Source: CAD feature listing. Evaluate the final solid. Frame: model axes, mm. A direction names the side the tool comes from. Coordinates: 2 decimals unless noted, no trailing zeros. Write each loop counter-clockwise with the first axis right and the second up, starting at its lowest first coordinate (ties: lowest second). Pieces come first, ordered by that corner, then holes. Notation, with made-up numbers: M 86,49 L 123,49 A24 ccw 123,64 Z; hole C 27.5,15 d2. An arc over 180 degrees is marked long. One line per item, written item: value. Start each with the question number.
Item 1: Cut plane B-B, the plane z = 39. Output: boundary loops of the cut face in (x, y) (3 decimals), then the cut area to 3 significant figures.
Item 2: Ray query, L1, parallel to X at y = 44, z = 7.5 (1 decimal); L2, parallel to X at y = 31, z = 8 (1 decimal); L3, parallel to Y at x = 54.5, z = 28.5 (3 decimals). Return the intervals inside material, ascending. Write a range as from..to.
Item 3: Mould query, pull axis X, two halves, no side actions, for faces 3 (the flat face through (54.153, 67, 8)), 4 (the flat face through (72.758, 93.034, -1.212)), 5 (the flat face through (31.75, 96, 20)). Classes: released by +X, released by -X, zero draft, split by the parting line, or undercut.
Item 4: Cut plane C-C, the plane y = 11. Output: boundary loops of the cut face in (x, z) (1 decimal), then the cut area to 3 significant figures.
Item 5: Pin query (flat end, axial travel): P1, Ø21.5, axis at x = 25.5, z = 22, coming from the +Y side; P2, Ø5, axis at x = 13.5, z = 26, coming from the -Y side; P3, Ø0.5, axis at x = 8, y = 82.5, coming from the +Z side; P4, Ø12, axis at x = 35, z = 4.5, coming from the +Y side (3 decimals). Return the tip coordinate at first contact, or that it passes through.
Item 6: Set-up query: faces 1 (the flat face through (54.4, 72.4, 15.24)), 2 (the cylindrical face through (37.591, 103.504, 19.678)). Return all of +Z, -Z, +X, -X, +Y, -Y with unobstructed straight access to the full face (end or side cutting, diameter ignored); none if empty.
Item 7: Cut plane D-D, the plane y = 46.5. Output: boundary loops of the cut face in (x, z) (1 decimal).
```python
from build123d import *

# Parameters (mm, degrees)
SKETCH1_R           = 2.54
BOSS_EXTRUDE1_DEPTH = 3.175
SKETCH1_3_W         = 13.97
SKETCH1_3_H         = 1.5875
BOSS_EXTRUDE2_DEPTH = 10.16
SKETCH1_4_R         = 2.54
BOSS_EXTRUDE3_DEPTH = 43.18
SKETCH2_W           = 13.97
SKETCH2_H           = 1.5875
BOSS_EXTRUDE4_DEPTH = 15.24
SKETCH3_R           = 8.255
CUT_EXTRUDE1_DEPTH  = 15.24
CHAMFER1_SIZE       = 3.175


with BuildPart() as part:
    # Sketch1 → Boss-Extrude1 (new body)
    with BuildSketch(Plane.XY):
        with BuildLine():
            Line((0, 0), (31.75, 0))
            Line((31.75, 0), (31.75, -2.54))
            ThreePointArc((31.75, -2.54), (37.465, -8.255), (43.18, -2.54))
            Line((43.18, -2.54), (43.18, 0))
            Line((43.18, 0), (74.93, 0))
            Line((74.93, 0), (74.93, 95.25))
            Line((74.93, 95.25), (43.18, 95.25))
            Line((43.18, 95.25), (43.18, 97.79))
            ThreePointArc((43.18, 97.79), (37.465, 103.505), (31.75, 97.79))
            Line((31.75, 97.79), (31.75, 95.25))
            Line((31.75, 95.25), (0, 95.25))
            Line((0, 95.25), (0, 0))
        make_face()
        with Locations((37.465, -2.54)):
            Circle(SKETCH1_R, mode=Mode.SUBTRACT)
        with Locations((37.465, 97.79)):
            Circle(SKETCH1_R, mode=Mode.SUBTRACT)
    extrude(amount=-BOSS_EXTRUDE1_DEPTH)

    # Sketch1_3 → Boss-Extrude2 (add)
    with BuildSketch(Plane.XY):
        Polygon((43.815, 9.525), (43.815, 75.5015), (29.845, 75.5015), (29.845, 77.089), (43.815, 77.089), (45.4025, 77.089), (45.4025, 3.175), (43.815, 3.175), (43.815, 7.9375), (3.175, 7.9375), (3.175, 9.525), align=None)
        with Locations((10.16, 76.29525)):
            Rectangle(SKETCH1_3_W, SKETCH1_3_H)
    extrude(amount=BOSS_EXTRUDE2_DEPTH)

    # Sketch1_4 → Boss-Extrude3 (add)
    with BuildSketch(Plane.XY):
        with BuildLine():
            Line((0, 95.25), (0, 0))
            Line((0, 0), (31.75, 0))
            Line((31.75, 0), (31.75, -2.54))
            ThreePointArc((31.75, -2.54), (37.465, -8.255), (43.18, -2.54))
            Line((43.18, -2.54), (43.18, 0))
            Line((43.18, 0), (74.93, 0))
            Line((74.93, 0), (74.93, 95.25))
            Line((74.93, 95.25), (43.18, 95.25))
            Line((43.18, 95.25), (43.18, 97.79))
            ThreePointArc((43.18, 97.79), (37.465, 103.505), (31.75, 97.79))
            Line((31.75, 97.79), (31.75, 95.25))
            Line((31.75, 95.25), (0, 95.25))
        make_face()
        with Locations((37.465, -2.54)):
            Circle(SKETCH1_4_R, mode=Mode.SUBTRACT)
        Polygon((3.175, 7.9375), (3.175, 9.525), (3.175, 75.5015), (3.175, 77.089), (3.175, 92.075), (71.755, 92.075), (71.755, 3.175), (45.4025, 3.175), (43.815, 3.175), (3.175, 3.175), align=None, mode=Mode.SUBTRACT)
        with Locations((37.465, 97.79)):
            Circle(SKETCH1_4_R, mode=Mode.SUBTRACT)
    extrude(amount=BOSS_EXTRUDE3_DEPTH)

    # Sketch2 → Boss-Extrude4 (add)
    with BuildSketch(Plane.XY):
        with Locations((10.16, 82.20075)):
            Rectangle(SKETCH2_W, SKETCH2_H)
        Polygon((54.737, 82.9945), (55.740027204, 82.9945), (55.740027204, 52.60975), (54.152527204, 52.60975), (54.152527204, 81.407), (29.845, 81.407), (29.845, 82.9945), align=None)
        Polygon((54.152527204, 3.175), (55.740027204, 3.175), (55.740027204, 33.55975), (54.152527204, 33.55975), (54.152527204, 9.525), (3.175, 9.525), (3.175, 7.9375), (54.152527204, 7.9375), align=None)
    extrude(amount=BOSS_EXTRUDE4_DEPTH)

    # Sketch3 → Cut-Extrude1 (cut)
    with BuildSketch(Plane.ZY.offset(-71.755)):
        with Locations((27.1145, 13.462)):
            Circle(SKETCH3_R)
    extrude(amount=-CUT_EXTRUDE1_DEPTH, mode=Mode.SUBTRACT)

    # Chamfer1
    chamfer1_edges = [part.edges().sort_by_distance(p)[0] for p in [
        (0, 0, 20.0025),
        (0, 95.25, 20.0025),
        (59.055, 0, -3.175),
        (74.93, 95.25, 20.0025),
        (74.93, 0, 20.0025),
        (74.93, 47.625, -3.175),
        (59.055, 95.25, -3.175),
        (15.875, 95.25, -3.175),
        (0, 47.625, -3.175),
        (15.875, 0, -3.175),
    ]]
    chamfer(chamfer1_edges, length=CHAMFER1_SIZE)


solid = part.part
```
From the geometry:
1. outline: M 0,3.175 L 3.175,0 L 31.75,0 L 31.75,-2.54 A5.715 ccw 43.18,-2.54 L 43.18,0 L 71.755,0 L 74.93,3.175 L 74.93,92.075 L 71.755,95.25 L 43.18,95.25 L 43.18,97.79 A5.715 ccw 31.75,97.79 L 31.75,95.25 L 3.175,95.25 L 0,92.075 Z; hole M 3.175,3.175 L 71.755,3.175 L 71.755,92.075 L 3.175,92.075 Z; hole C 37.465,-2.54 d5.08; hole C 37.465,97.79 d5.08
1. area: 1,140 mm²
2. L1: x = 0..3.2, 43.8..45.4, 71.8..74.9
2. L2: x = 0..3.2, 43.8..45.4, 54.2..55.7, 71.8..74.9
2. L3: y = 0..3.175, 92.075..95.25
3. face 3: undercut
3. face 4: released by +X
3. face 5: released by -X
4. outline: M 0,0 L 3.2,-3.2 L 71.8,-3.2 L 74.9,0 L 74.9,19.2 L 71.8,19.2 L 71.8,0 L 55.7,0 L 55.7,15.2 L 54.2,15.2 L 54.2,0 L 45.4,0 L 45.4,10.2 L 43.8,10.2 L 43.8,0 L 3.2,0 L 3.2,43.2 L 0,43.2 Z; M 71.8,35 L 74.9,35 L 74.9,43.2 L 71.8,43.2 Z
4. area: 492 mm²
5. P1: stops at y = 103.37
5. P2: stops at y = 0
5. P3: stops at z = 15.24
5. P4: stops at y = 103.505
6. face 1: +Z
6. face 2: +Z, -Z, +Y
7. outline: M 0,0 L 3.2,-3.2 L 71.8,-3.2 L 74.9,0 L 74.9,43.2 L 71.8,43.2 L 71.8,0 L 45.4,0 L 45.4,10.2 L 43.8,10.2 L 43.8,0 L 3.2,0 L 3.2,43.2 L 0,43.2 Z
